Geometry check sheet. Reference: drawing and pictorial views, mm from the part's lowest x, y, z. A direction names the side the tool comes from. Give positions to 0.01 mm unless a question says otherwise; leave off trailing zeros. Loops run counter-clockwise (first coordinate to the right, second up) from the corner with the lowest first, then second, coordinate; pieces in that order, holes last. Notation, with made-up numbers: (35.5, -1) - (66.5, -1) arc R19 ccw to (66.5, 24) - close; hole circle Ø8 at (67, 28). An arc over 180 degrees is marked (long way). Answer in a Markdown table with one row per item. Add a question column.
(1) Go/stop test with flat-tipped pins: P1, Ø4, axis at x = 66, z = 49, coming from the +Y side; P2, Ø23, axis at x = 37, y = 23.5, coming from the +Z side; P3, Ø3, axis at y = 22, z = 44.5, coming from the +X side; P4, Ø4, axis at x = 10, z = 7.5, coming from the +Y side. Record where each tip stops, or that it passes through.
(2) Sectioned sample at C-C on z = 22. Enter the section's corners in (x, y).
(3) Draft check along Z on the marked faces 1 and 2. Enter one of: released by +Z, released by -Z, zero draft, split by the parting line, or undercut.
(4) Sectioned sample at B-B on x = 90. Enter the section's corners in (y, z).
(5) Sectioned sample at A-A on y = 16. Enter the section's corners in (x, z), then the cut area to 3 significant figures.
(6) Sectioned sample at D-D on x = 63.5. Enter the section's corners in (y, z).
(7) Thickness scan on L1, parallel to X at y = 3.15, z = 7.5; L2, parallel to Z at x = 4.5, y = 23; L3, parallel to Y at x = 3.5, z = 45.25. Record the ranges inside material, lowest first.
(8) Set-up check for the marked faces 3 and 4: record each of +Z, -Z, +X, -X, +Y, -Y from which the full face is reachable in a straight line by a thin tool's end or side.
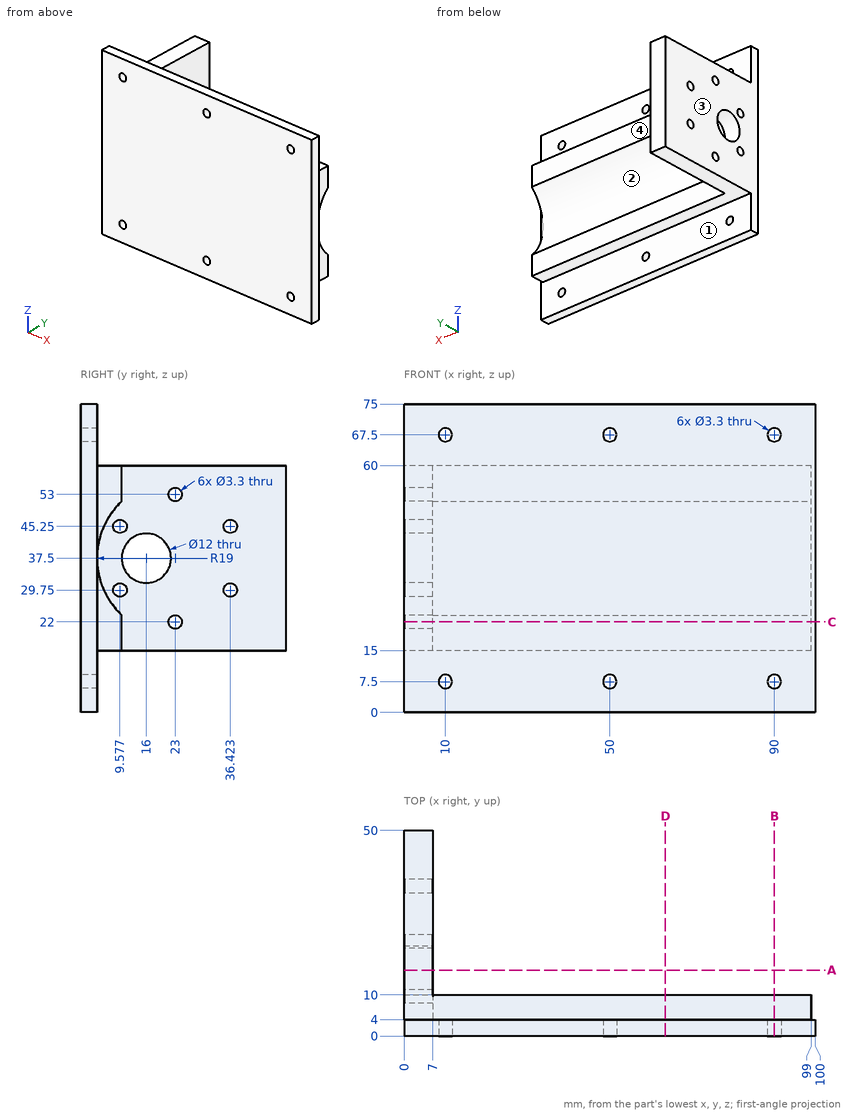
Reply:
| question | item | result |
|---|---|---|
| 1 | P1 | y = 9.63 |
| 1 | P2 | through |
| 1 | P3 | x = 7 |
| 1 | P4 | y = 4 |
| 2 | outline | (0, 0) - (100, 0) - (100, 4) - (99, 4) - (99, 10) - (7, 10) - (7, 21.35) - (0, 21.35) - close; (0, 24.65) - (7, 24.65) - (7, 50) - (0, 50) - close |
| 3 | face 1 | zero draft |
| 3 | face 2 | undercut |
| 4 | outline | (0, 0) - (4, 0) - (4, 5.85) - (0, 5.85) - close; (0, 9.15) - (4, 9.15) - (4, 15) - (10, 15) - (10, 23.64) arc R19 cw to (10, 51.36) - (10, 60) - (4, 60) - (4, 65.85) - (0, 65.85) - close; (0, 69.15) - (4, 69.15) - (4, 75) - (0, 75) - close |
| 5 | outline | (0, 15) - (7, 15) - (7, 31.5) - (0, 31.5) - close; (0, 43.5) - (7, 43.5) - (7, 60) - (0, 60) - close |
| 5 | area | 231 mm^2 |
| 6 | outline | (0, 0) - (4, 0) - (4, 15) - (10, 15) - (10, 23.64) arc R19 cw to (10, 51.36) - (10, 60) - (4, 60) - (4, 75) - (0, 75) - close |
| 7 | L1 | 0 to 8.35, 11.65 to 48.35, 51.65 to 88.35, 91.65 to 100 |
| 7 | L2 | 15 to 20.35, 23.65 to 51.35, 54.65 to 60 |
| 7 | L3 | 0 to 7.93, 11.23 to 34.77, 38.07 to 50 |
| 8 | face 3 | +Z, -Z, -X, +Y, -Y |
| 8 | face 4 | +Z, -Z, +X, +Y |
